from build123d import *

# Parameters (mm, degrees)
F0_W     = 139.2736807466
F0_H     = 131.1470270157
F1_DEPTH = 101.6
F2_T     = -2.54
F4_DEPTH = 25.4


with BuildPart() as f1:
    # F0 (on Top) → F1 (new body)
    with BuildSketch(Plane.XY):
        with Locations((-2.6764906943, 1.5565976501)):
            Rectangle(F0_W, F0_H)
    extrude(amount=F1_DEPTH)

    # F2
    f2_openings = [f1.faces().sort_by_distance(p)[0] for p in [
        (-2.676491, 1.556598, 101.6),
    ]]
    offset(amount=F2_T, openings=f2_openings)

    # F3 (on face) → F4 (join)
    with BuildSketch(Plane.XZ.offset(-64.5901111579)):
        with BuildLine():
            Line((-69.7733310676, 101.6), (-25.7274541641, 101.6))
            ThreePointArc((-25.7274541641, 101.6), (-86.7891143722, 108.0409788687), (-69.7733310676, 49.0454224709))
            Line((-69.7733310676, 49.0454224709), (-69.7733310676, 101.6))
        make_face()
        with BuildLine():
            ThreePointArc((-69.7733310676, 49.0454224709), (-36.6361593712, 54.3579049697), (-21.4188937376, 84.2699334025))
            ThreePointArc((-21.4188937376, 84.2699334025), (-22.5121831898, 93.1987477306), (-25.7274541641, 101.6))
            Line((-25.7274541641, 101.6), (-69.7733310676, 101.6))
            Line((-69.7733310676, 101.6), (-69.7733310676, 49.0454224709))
        make_face()
    extrude(amount=F4_DEPTH)


solid = f1.part
Verification items for the finished model (mm, model axes). A direction names the side the tool comes from. Coordinates: 2 decimals unless noted, no trailing zeros. Write each loop counter-clockwise with the first axis right and the second up, starting at its lowest first coordinate (ties: lowest second). Pieces come first, ordered by that corner, then holes. Notation, with made-up numbers: M 5.5,33.25 L 55.5,33.25 A10 cw 55.5,37.25 Z; hole C 4.25,-0.75 d5. An arc over 180 degrees is marked long. One line per question, with ' | ' between items.
1) Release check for a two-part mould opening along Y. For faces 1 (the face through (-4, 2, 2.54)), 2 (the face through (64.42, 1, 51)), 3 (the face through (-4, 67.13, 50)), 4 (the face through (-4, -64.017, 50)) record: +Y half, -Y half, draft (parallel to the pull), parting line (faces both ways), or undercut.
Solutions:
face 1: undercut | face 2: undercut | face 3: +Y half | face 4: -Y half
2) Sectioned sample at A-A on z = 43. Record the cut outline in (x, y).
Solutions:
outline: M -72.31,-64.02 L 66.96,-64.02 L 66.96,67.13 L -72.31,67.13 Z; hole M -69.77,-61.48 L 64.42,-61.48 L 64.42,64.59 L -69.77,64.59 Z
3) Access from +Z, -Z, +X, -X, +Y, -Y to the whole of each face (thin tool, end or side, straight path). Record for faces 5 (the face through (11, 64.59, 51)), 6 (the face through (66.96, 1, 50)), 7 (the face through (-4, -61.477, 51)).
Solutions:
face 5: none | face 6: +Z, -Z, +X, +Y, -Y | face 7: +Z
4) Depth check by flat-ended pin: pin 1 Ø6 at (x, y) = (-32.5, -45.5) entering from -Z; pin 2 Ø1 at (y, z) = (-20, 74) entering from -X; pin 3 Ø3 at (x, y) = (18, 29.5) entering from +Z. Enter the tip coordinate at first touch or a pass-through.
Solutions:
pin 1: z = 0 | pin 2: x = -72.31 | pin 3: z = 2.54
5) Sectioned sample at C-C on y = 2.5. Record the cut outline in (x, z), then the cut area to 3 significant figures.
Solutions:
outline: M -72.31,0 L 66.96,0 L 66.96,101.6 L 64.42,101.6 L 64.42,2.54 L -69.77,2.54 L -69.77,101.6 L -72.31,101.6 Z | area: 857 mm^2
6) Sectioned sample at B-B on x = 38. Record the cut outline in (y, z).
Solutions:
outline: M -64.02,0 L 67.13,0 L 67.13,101.6 L 64.59,101.6 L 64.59,2.54 L -61.48,2.54 L -61.48,101.6 L -64.02,101.6 Z
7) Material ranges on L1, parallel to X at y = 57.5, z = 41.5; L2, parallel to Y at x = -10.5, z = 69; L3, parallel to Y at x = -50.5, z = 84, recorded low to high.
Solutions:
L1: -72.31 to -69.77, 64.42 to 66.96 | L2: -64.02 to -61.48, 64.59 to 67.13 | L3: -64.02 to -61.48, 39.19 to 67.13
8) Sectioned sample at D-D on z = 70. Record the cut outline in (x, y), then the cut area to 3 significant figures.
Solutions:
outline: M -92.57,39.19 L -72.31,39.19 L -72.31,-64.02 L 66.96,-64.02 L 66.96,67.13 L -72.31,67.13 L -72.31,64.59 L -92.57,64.59 Z; hole M -69.77,-61.48 L 64.42,-61.48 L 64.42,64.59 L -24.28,64.59 L -24.28,39.19 L -69.77,39.19 Z | area: 3,020 mm^2
